Here's how the part is built. I have some questions about the finished solid (model axes, mm). A direction names the side the tool comes from. Give positions to 0.01 mm unless a question says otherwise; leave off trailing zeros. Order: outer loops, then holes, each group sorted by start corner. A loop starts at its lowest first (then second) coordinate and runs counter-clockwise, first axis right, second up.
Autodesk Inventor part; units mm, degrees
ref_plane "Work Plane3" through (0, 0, 5) normal (0, 0, 1) x (1, 0, 0)
ref_plane "Work Plane4" through (0, 0, 12) normal (0, 0, 1) x (1, 0, 0)
ref_plane "YZ Plane" through (0, 0, 0) normal (1, 0, 0) x (0, 1, 0)
sketch "Sketch1" plane through (0, 0, 0) normal (0, 0, 1) x (1, 0, 0)
  circle A0 centre (0, 0) radius 26
  dimension "d0" = 52
extrude "Extrusion1" add sketch "Sketch1" along normal blind 5
chamfer "Chamfer2" distance 2 angle 45 1 edges at (-26, 0, 5)
ref_plane "Work Plane3" through (0, 0, 5) normal (0, 0, 1) x (1, 0, 0)
sketch "Sketch3" plane through (0, 0, 5) normal (0, 0, 1) x (1, 0, 0)
  circle A0 centre (0, 0) radius 12.5
  dimension "d6" = 25
extrude "Extrusion2" add sketch "Sketch3" along normal blind 7
ref_plane "Work Plane4" through (0, 0, 12) normal (0, 0, 1) x (1, 0, 0)
sketch "Sketch4" plane through (0, 0, 12) normal (0, 0, 1) x (1, 0, 0)
  circle A0 centre (0, 0) radius 8
  dimension "d9" = 16
extrude "Extrusion3" cut sketch "Sketch4" against normal blind 12
sketch "Sketch2" plane through (0, 0, 0) normal (0, 0, -1) x (-1, 0, 0)
  line L0 (0, 0) -> (-23.1702, 23.1702)
  line L1 (0, 0) -> (32.7676, 0) construction
  line L2 (-23.1702, 23.1702) -> (18.3848, -18.3848)
  circle A0 centre (0, 0) radius 26
  line L3 (0, 0) -> (-21.488, -21.488)
  line L4 (0, 0) -> (30.3887, 0) construction
  line L5 (-21.488, -21.488) -> (18.3848, 18.3848)
  circle A1 centre (0, 0) radius 8
  line L6 (0, 8) -> (0, 17)
  circle A2 centre (0, 17) radius 3
  line L7 (0, -26) -> (0, 26)
  circle A3 centre (-14.7224, -8.5) radius 3
  circle A4 centre (14.7224, -8.5) radius 3
  dimension "d4" = 135
  dimension "d5" = 135
  dimension "d19" = 9
  dimension "d20" = 6
  dimension "d23" = 360
extrude "Extrusion4" cut sketch "Sketch2" against normal blind 12 contours A2 L7 L6 | L6 L7 A2 | A3 | A4
properties part number "EndBush" material "Titanium"
Q1. If we section it at D-D on z = 11.25: List the corners of the cut face in (x, y) for me.
Filled sheet:
outline: circle Ø25 at (0, 0); hole circle Ø16 at (0, 0)
Q2. Thinking about a two-plate mould opening in Y: for faces 3 (the face through (-6.14, -5.41, 0)), 4 (the face through (-20.633, 15.821, 1.479)), 5 (the face through (17.72, -8.37, 2.46)), which applies, released by +Y, released by -Y, zero draft, split by the parting line, or undercut?
Filled sheet:
face 3: zero draft
face 4: split by the parting line
face 5: undercut
Q3. For faces 1 (the face through (11.923, -3.755, 8.451)), 2 (the face through (0.65, 14.07, 2.46)), which set-ups out of +Z, -Z, +X, -X, +Y, -Y let a thin tool reach every point of the face, with its end or its side?
Filled sheet:
face 1: +Z
face 2: +Z, -Z
Q4. If we section it at A-A on x = 0: List the corners of the cut face in (y, z) for me, plus the area to 3 significant figures.
Filled sheet:
outline: (-26, 0) - (-8, 0) - (-8, 12) - (-12.5, 12) - (-12.5, 5) - (-24, 5) - (-26, 3) - close; (8, 0) - (14, 0) - (14, 5) - (12.5, 5) - (12.5, 12) - (8, 12) - close; (20, 0) - (26, 0) - (26, 3) - (24, 5) - (20, 5) - close
area: 209 mm2
Q5. I'm going to push flat-ended pins straight in: P1, Ø1, axis at y = -2, z = 6.5, coming from the +X side; P2, Ø3, axis at y = -9.5, z = 5.5, coming from the +X side; P3, Ø3, axis at x = -9.5, y = -17.5, coming from the +Z side. Where does each tip first touch, or does it pass through?
Filled sheet:
P1: stops at x = 12.41
P2: stops at x = 23.23
P3: stops at z = 5
Q6. If we section it at C-C on z = 2: List the corners of the cut face in (x, y) for me.
Filled sheet:
outline: circle Ø52 at (0, 0); hole circle Ø6 at (-14.72, -8.5); hole circle Ø16 at (0, 0); hole circle Ø6 at (0, 17); hole circle Ø6 at (14.72, -8.5)
Q7. I need wall thicknesses on L1, parallel to X at y = -10, z = 3.25; L2, parallel to Y at x = 0, z = 8; L3, parallel to X at y = -7, z = 2.5. Which ranges of each line are inside material? Lowest first, please.
Filled sheet:
L1: x = -23.73 to -17.32, -12.12 to 12.12, 17.32 to 23.73
L2: y = -12.5 to -8, 8 to 12.5
L3: x = -25.04 to -17.32, -12.12 to -3.87, 3.87 to 12.12, 17.32 to 25.04
Q8. If we section it at B-B on y = 0: List the corners of the cut face in (x, z) for me, plus the area to 3 significant figures.
Filled sheet:
outline: (-26, 0) - (-8, 0) - (-8, 12) - (-12.5, 12) - (-12.5, 5) - (-24, 5) - (-26, 3) - close; (8, 0) - (26, 0) - (26, 3) - (24, 5) - (12.5, 5) - (12.5, 12) - (8, 12) - close
area: 239 mm2
